Drawing for the job (mm, zero at the part's lowest x, y, z). A direction names the side the tool comes from. Give positions to 0.01 mm unless a question says otherwise; leave off trailing zeros. Order: outer loops, then holes, each group sorted by start corner. A loop starts at its lowest first (then second) coordinate and runs counter-clockwise, first axis right, second up. Notation, with made-up numbers: (27.5, -8.5) - (37.5, -8.5) arc R24 ccw to (37.5, 10.5) - close; hole circle Ø2 at (-26.5, -16). An arc over 180 degrees is marked (long way). Use a Markdown table: item, result.
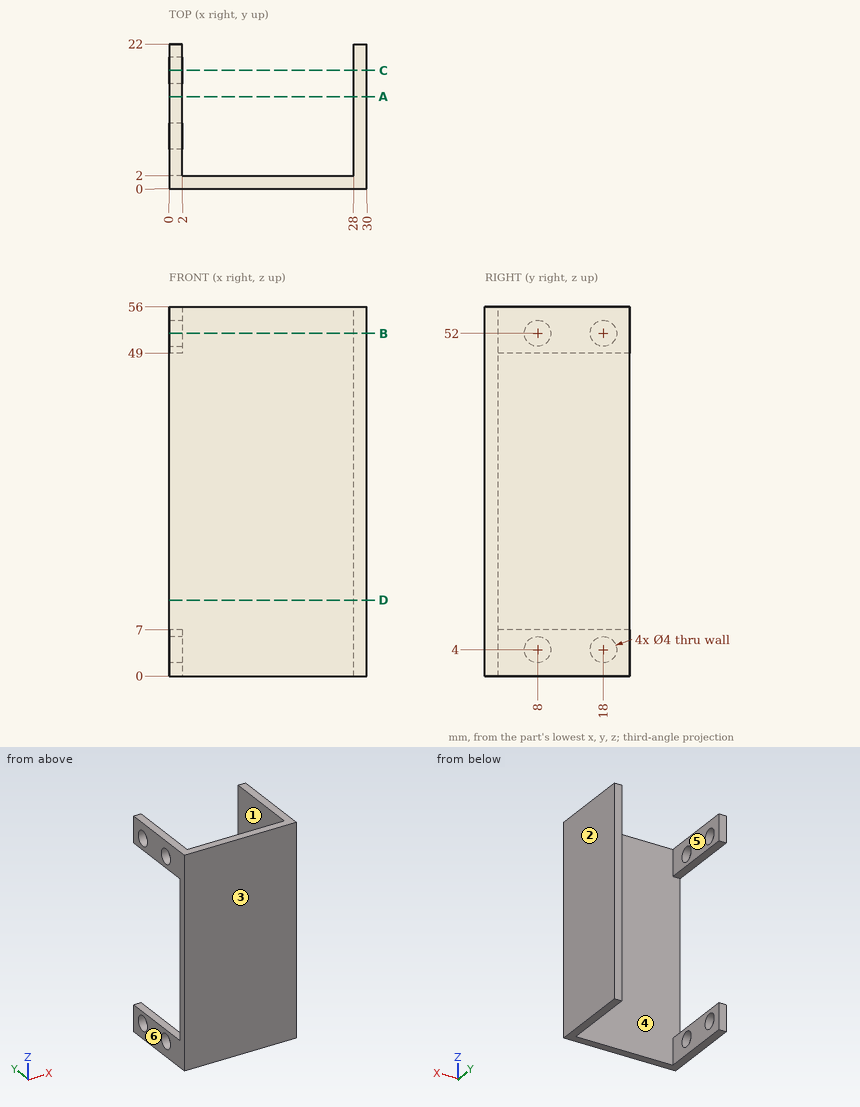
1) Wall check: line 1 (Y direction, x = 1.45, z = 52); line 2 (Y direction, x = 23, z = 34); line 3 (X direction, y = 13.5, z = 32). Give the ranges that are in metal, low to high. Write a range as from..to.
Computed:
| item | result |
|---|---|
| line 1 | y = 0..6, 10..16, 20..22 |
| line 2 | y = 0..2 |
| line 3 | x = 28..30 |
2) Two-plate mould, pull along X, no slides. Class the marked faces 3, 4, 5 and 6: +X half, -X half, draft (parallel to the pull), parting line (faces both ways), or undercut.
Computed:
| item | result |
|---|---|
| face 3 | draft |
| face 4 | undercut |
| face 5 | undercut |
| face 6 | -X half |
3) Slice it at D-D (z = 11.5). Write the cut outline in (x, y), and give its area (3 significant figures).
Computed:
| item | result |
|---|---|
| outline | (0, 0) - (30, 0) - (30, 22) - (28, 22) - (28, 2) - (0, 2) - close |
| area | 100 mm² |
4) Pin check, flat tips, straight feed: P1, Ø1, axis at x = 9.5, z = 45.5, coming from the +Y side; P2, Ø3.5, axis at y = 8, z = 52, coming from the -X side. Stop position of each tip, or through.
Computed:
| item | result |
|---|---|
| P1 | stops at y = 2 |
| P2 | stops at x = 28 |
5) Slice it at C-C (y = 18). Write the cut outline in (x, z).
Computed:
| item | result |
|---|---|
| outline | (0, 0) - (2, 0) - (2, 2) - (0, 2) - close; (0, 6) - (2, 6) - (2, 7) - (0, 7) - close; (0, 49) - (2, 49) - (2, 50) - (0, 50) - close; (0, 54) - (2, 54) - (2, 56) - (0, 56) - close; (28, 0) - (30, 0) - (30, 56) - (28, 56) - close |
6) Slice it at B-B (z = 52). Write the cut outline in (x, y), and give its area (3 significant figures).
Computed:
| item | result |
|---|---|
| outline | (0, 0) - (30, 0) - (30, 22) - (28, 22) - (28, 2) - (2, 2) - (2, 6) - (0, 6) - close; (0, 10) - (2, 10) - (2, 16) - (0, 16) - close; (0, 20) - (2, 20) - (2, 22) - (0, 22) - close |
| area | 124 mm² |
7) Slice it at A-A (y = 14). Write the cut outline in (x, z), and give its area (3 significant figures).
Computed:
| item | result |
|---|---|
| outline | (0, 0) - (2, 0) - (2, 7) - (0, 7) - close; (0, 49) - (2, 49) - (2, 56) - (0, 56) - close; (28, 0) - (30, 0) - (30, 56) - (28, 56) - close |
| area | 140 mm² |
8) Tool access for the marked faces 1 and 2: list every direction of +Z, -Z, +X, -X, +Y, -Y with a clear straight run to the whole face (end or side of a thin tool).
Computed:
| item | result |
|---|---|
| face 1 | +Z, -Z, +Y |
| face 2 | +Z, -Z, +X, +Y, -Y |
